Source: CAD feature listing. Evaluate the final solid. Frame: model axes, mm. A direction names the side the tool comes from. Round coordinates to 2 decimals unless told otherwise and drop trailing zeros. Order: outer loops, then holes, each group sorted by start corner. A loop starts at its lowest first (then second) coordinate and runs counter-clockwise, first axis right, second up. Notation, with made-up numbers: (61, 39) -> (83, 39) arc R19 ccw to (83, 63) -> close; hole circle Ø9 at (-19.5, 82.5). An arc over 180 degrees is marked (long way). One line per item, written item: value. Start each with the question number.
1) Section B-B (y = -19). Return the cut outline in (x, z).
2) Reachability of faces 4 (the face through (-55, 1, 8)), 5 (the face through (-51, 71.314, 10)) from +Z, -Z, +X, -X, +Y, -Y: full face, straight path, thin tool, end or side. Return the list, or none.
3) Section A-A (x = -12.5). Return the cut outline in (y, z), and give its area (3 significant figures).
4) Pin query (flat end, axial travel): P1, Ø3, axis at x = 22, y = -63.5, coming from the +Z side; P2, Ø0.6, axis at x = 52.5, y = -75.5, coming from the +Z side; P3, Ø0.9, axis at x = -51, z = 10.5, coming from the +Y side. Return the tip coordinate at first contact, or that it passes through.
5) Ray query, L1, parallel to Y at x = 44, z = 6; L2, parallel to X at y = -24, z = 13; L3, parallel to Y at x = 52.5, z = 16.4. Return the intervals inside material, ascending.
6) Mould query, pull axis Y, two halves, no side actions, for faces 1 (the face through (1, 75, 10)), 2 (the face through (55, -1, 8)), 3 (the face through (53, -79, 9)). Classes: pulls with the +Y half, pulls with the -Y half, needs draft (parallel to the pull), parting line crosses it, or undercut.
7) Section C-C (z = 12.25). Return the cut outline in (x, y), and give its area (3 significant figures).
Solid Edge part; units mm, degrees
sketch "Sketch1" plane through (0, 0, 0) normal (0, 0, 1) x (1, 0, 0)
  line L0 (55, -80) -> (55, 80)
  line L1 (55, 80) -> (-55, 80)
  line L2 (-55, 80) -> (-55, -80)
  line L3 (-55, -80) -> (55, -80)
extrude "ExtrudedProtrusion_2" add sketch "Sketch1" along normal blind 17
fillet "Round_3" radius 5 4 edges at (-55, 80, 8.5) (55, 80, 8.5) (55, -80, 8.5) (-55, -80, 8.5)
sketch "Sketch2" plane through (0, 0, 17) normal (0, 0, 1) x (1, 0, 0)
  line L0 (50, -75) -> (50, 75)
  line L1 (50, 75) -> (-50, 75)
  line L2 (-50, 75) -> (-50, -75)
  line L3 (-50, -75) -> (50, -75)
extrude "ExtrudedCutout_1" cut sketch "Sketch2" against normal blind 15
sketch "Sketch3" plane through (0, 0, 17) normal (0, 0, 1) x (1, 0, 0)
  circle A0 centre (-52.5, 75) radius 1
  circle A1 centre (52.5, 75) radius 1
  circle A2 centre (52.5, 0) radius 1
  circle A3 centre (52.5, -75) radius 1
  circle A4 centre (-52.5, -75) radius 1
  circle A5 centre (-52.5, 0) radius 1
extrude "ExtrudedCutout_2" cut sketch "Sketch3" against normal blind 1
sketch "Sketch4" plane through (0, 0, 17) normal (0, 0, 1) x (1, 0, 0)
  line L0 (-53, 71.3143) -> (-53, 51.3143)
  line L1 (-53, 51.3143) -> (-53, 41.3143)
  line L2 (-53, 41.3143) -> (-50, 41.3143)
  line L3 (-50, 41.3143) -> (-50, 71.3143)
  line L4 (-50, 71.3143) -> (-53, 71.3143)
extrude "ExtrudedCutout_3" cut sketch "Sketch4" against normal blind 15
Findings:
1. outline: (-55, 0) -> (55, 0) -> (55, 17) -> (50, 17) -> (50, 2) -> (-50, 2) -> (-50, 17) -> (-55, 17) -> close
2. face 4: +Z, -Z, -X, +Y, -Y
2. face 5: +Z
3. outline: (-80, 0) -> (80, 0) -> (80, 17) -> (75, 17) -> (75, 2) -> (-75, 2) -> (-75, 17) -> (-80, 17) -> close
3. area: 470 mm2
4. P1: z = 2
4. P2: z = 16
4. P3: y = 79.97
5. L1: -80 to -75, 75 to 80
5. L2: -55 to -50, 50 to 55
5. L3: -79.33 to -76, -74 to -1, 1 to 74, 76 to 79.33
6. face 1: undercut
6. face 2: needs draft
6. face 3: pulls with the -Y half
7. outline: (-55, -75) arc R5 ccw to (-50, -80) -> (50, -80) arc R5 ccw to (55, -75) -> (55, 75) arc R5 ccw to (50, 80) -> (-50, 80) arc R5 ccw to (-55, 75) -> close; hole (-53, 41.31) -> (-50, 41.31) -> (-50, -75) -> (50, -75) -> (50, 75) -> (-50, 75) -> (-50, 71.31) -> (-53, 71.31) -> close
7. area: 2,490 mm2
